from build123d import *

# Parameters (mm, degrees)
SKETCH1_W           = 50
SKETCH1_H           = 25
BOSS_EXTRUDE1_DEPTH = 3
SKETCH3_W           = 50
SKETCH3_H           = 2
BOSS_EXTRUDE2_DEPTH = 15
SKETCH5_R           = 1.25
CUT_EXTRUDE1_DEPTH  = 15
SKETCH6_R           = 1.75
CUT_EXTRUDE2_DEPTH  = 15


with BuildPart() as part:
    # Sketch1 → Boss-Extrude1 (new body)
    with BuildSketch(Plane.XY):
        with Locations((-25, 12.5)):
            Rectangle(SKETCH1_W, SKETCH1_H)
    extrude(amount=BOSS_EXTRUDE1_DEPTH)

    # Sketch3 → Boss-Extrude2 (add)
    with BuildSketch(Plane.XY.offset(3)):
        with Locations((-25, 24)):
            Rectangle(SKETCH3_W, SKETCH3_H)
    extrude(amount=BOSS_EXTRUDE2_DEPTH)

    # Sketch5 → Cut-Extrude1 (cut)
    with BuildSketch(Plane.XY.offset(3)):
        with Locations((-46.500140762, 20.00924034)):
            Circle(SKETCH5_R)
        with Locations((-46.500140762, 3.00924034)):
            Circle(SKETCH5_R)
        with Locations((-3.500140762, 20.00924034)):
            Circle(SKETCH5_R)
        with Locations((-3.500140762, 3.00924034)):
            Circle(SKETCH5_R)
        with Locations((-3.500140762, 14.00924034)):
            Circle(SKETCH5_R)
        with Locations((-46.500140762, 14.00924034)):
            Circle(SKETCH5_R)
        with Locations((-3.500140762, 9.00924034)):
            Circle(SKETCH5_R)
        with Locations((-46.500140762, 9.00924034)):
            Circle(SKETCH5_R)
    extrude(amount=-CUT_EXTRUDE1_DEPTH, mode=Mode.SUBTRACT)

    # Sketch6 → Cut-Extrude2 (cut)
    with BuildSketch(Plane(origin=(0, 25, 0), x_dir=(1, 0, 0), z_dir=(0, 1, 0))):
        with Locations((-35.046148944, -11.535217426)):
            Circle(SKETCH6_R)
        with Locations((-15.046148944, -11.535217426)):
            Circle(SKETCH6_R)
    extrude(amount=-CUT_EXTRUDE2_DEPTH, mode=Mode.SUBTRACT)


solid = part.part
For this review, take the finished solid that the model builds, in its own axes (mm). A direction names the side the tool comes from. Give positions to 0.01 mm unless a question says otherwise; leave off trailing zeros. Order: outer loops, then holes, each group sorted by start corner. A loop starts at its lowest first (then second) coordinate and runs counter-clockwise, first axis right, second up. Notation, with made-up numbers: (19.25, 58.25) -> (62.25, 58.25) arc R14 cw to (62.25, 64.25) -> close; hole circle Ø7 at (80.25, -4.5). An arc over 180 degrees is marked (long way). Write item = value, one per line.
1) To check wall thickness, follow L1, parallel to Z at x = -45.5, y = 15; L2, parallel to Y at x = -22.5, z = 5.75. State the ranges of each line that lie inside material, in increasing order. Write a range as from..to.
Findings:
L1 = 0..3
L2 = 23..25
2) We need section B-B, the plane y = 2.25. Give the boundary of the cut face in (x, z).
Findings:
outline = (-50, 0) -> (-47.49, 0) -> (-47.49, 3) -> (-50, 3) -> close; (-45.51, 0) -> (-4.49, 0) -> (-4.49, 3) -> (-45.51, 3) -> close; (-2.51, 0) -> (0, 0) -> (0, 3) -> (-2.51, 3) -> close
3) For faces 1 (the face through (-25, 23, 10)), 2 (the face through (-45.345, 8.53, 1.521)), list the 3-axis set-ups (+Z, -Z, +X, -X, +Y, -Y) from which the entire face can be reached by the end or side of a thin tool; tool diameter is ignored.
Findings:
face_1 = +Z, +X, -X, -Y
face_2 = +Z, -Z
4) We need section A-A, the plane x = -16. Give the boundary of the cut face in (y, z), and give its area (3 significant figures).
Findings:
outline = (0, 0) -> (25, 0) -> (25, 10.07) -> (23, 10.07) -> (23, 3) -> (0, 3) -> close; (23, 13) -> (25, 13) -> (25, 18) -> (23, 18) -> close
area = 99.1 mm^2
5) Insertion check: pin 1 (2 mm diameter, centred on x = -6, z = 15.5, fed in from -Y); pin 2 (2 mm diameter, centred on x = -15.05, z = 11.54, fed in from -Y); pin 3 (11.5 mm diameter, centred on x = -23.5, y = 7.5, fed in from +Z); pin 4 (3 mm diameter, centred on x = -46.5, y = 20.01, fed in from -Z). Each pin has a flat end and moves straight along its axis. Give the tip position at first contact, or say it passes through.
Findings:
pin_1 = 23
pin_2 = through
pin_3 = 3
pin_4 = 0
6) We need section D-D, the plane x = -38. Give the boundary of the cut face in (y, z).
Findings:
outline = (0, 0) -> (25, 0) -> (25, 18) -> (23, 18) -> (23, 3) -> (0, 3) -> close
7) Draft analysis for pull direction Z (two halves, no side actions). For faces 3 (the face through (-3.77, 1.79, 1.52)), 4 (the face through (-25, 12, 3)), 5 (the face through (-33.43, 24.01, 12.21)), state which applies: pulls with the +Z half, pulls with the -Z half, needs draft (parallel to the pull), parting line crosses it, or undercut.
Findings:
face_3 = needs draft
face_4 = pulls with the +Z half
face_5 = undercut
8) We need section C-C, the plane z = 2.25. Count the separate pieces of the cut face and the enclosed holes in it, and give its area (3 significant figures).
Findings:
separate_pieces = 1
enclosed_holes = 8
area = 1,210 mm^2
